For this review, take the finished solid that the model builds, in its own axes (mm). Round coordinates to 2 decimals unless told otherwise and drop trailing zeros. Write each loop counter-clockwise with the first axis right and the second up, starting at its lowest first coordinate (ties: lowest second). Pieces come first, ordered by that corner, then holes. Notation, with made-up numbers: (83.5, 12.25) -> (110.5, 12.25) arc R22 cw to (110.5, 20.25) -> close; hole circle Ø3 at (74, 71). An arc over 180 degrees is marked (long way). Answer as CSV lines item,"result". Start each with the question number.
Item 1: Take a section at C-C on x = 59. Give the boundary of the cut face in (y, z).
Item 2: Take a section at B-B on x = 13. Give the boundary of the cut face in (y, z), then the cut area to 3 significant figures.
Item 3: Wall thickness on probe 1 along Y at (x, z) = (-12, -67); probe 2 along Z at (x, y) = (-73, -90); probe 3 along Z at (x, y) = (-70, -98): over which ranges is each line inside the solid? List them lowest first. Write a range as from..to.
Item 4: For pin 1 Ø8 at (y, z) = (-143, -89.5) entering from +X; pin 2 Ø2 at (x, y) = (-15, -198) entering from +Z; pin 3 Ø1.5 at (y, z) = (-196.5, -31) entering from +X, all flat-tipped, find the tip position at first contact; note any pin that passes through.
Item 5: Take a section at A-A on y = -196.5. Give the boundary of the cut face in (x, z).
```python
from build123d import *

# Parameters (mm, degrees)
F1_DEPTH = 254
F2_W     = 68.1403651834
F2_H     = 124.5979337706
F3_DEPTH = 50.8
F3_TAPER = -15


with BuildPart() as f1:
    # F0 (on Front) → F1 (new body)
    with BuildSketch(Plane.XZ):
        Polygon((-0.1336607501, -87.2124684732), (75.5950435996, 43.4904806316), (-75.4613828496, 43.7219878417), align=None)
    extrude(amount=F1_DEPTH)

    # F2 (on face) → F3 (join)
    with BuildSketch(Plane(origin=(-37.7975217998, 0, -21.7452403158), x_dir=(0, -1, 0), z_dir=(-0.8667906796, 0, -0.4986721545))):
        with Locations((122.2858987749, -13.2293350405)):
            Rectangle(F2_W, F2_H)
    extrude(amount=F3_DEPTH, taper=F3_TAPER)


solid = f1.part
```
Output values:
1,outline,"(-254, 14.85) -> (0, 14.85) -> (0, 43.52) -> (-254, 43.52) -> close"
2,outline,"(-254, -64.54) -> (0, -64.54) -> (0, 43.59) -> (-254, 43.59) -> close"
2,area,"27,500 mm^2"
3,probe 1,"y = -156.41..-88.16"
3,probe 2,"z = -62.43..17.93, 39.44..43.72"
3,probe 3,"z = -67.64..18.73, 34.23..43.71"
4,pin 1,"stops at x = 0.86"
4,pin 2,"stops at z = 43.63"
4,pin 3,"stops at x = 32.87"
5,outline,"(-75.46, 43.72) -> (-0.13, -87.21) -> (75.6, 43.49) -> close"
